Could you check a few things on this model? Use its own coordinates, in mm. Face numbers are marked on the shaded views. A direction names the side the tool comes from. Coordinates: 2 decimals unless noted, no trailing zeros. Loops run counter-clockwise (first coordinate to the right, second up) from the corner with the lowest first, then second, coordinate; pieces in that order, holes last.
from build123d import *

# Parameters (mm, degrees)
SKETCH001_R   = 8.9
SKETCH001_R_2 = 7.9
PAD001_DEPTH  = 10
SKETCH002_W   = 2.5
SKETCH002_H   = 12
PAD002_DEPTH  = 2
SKETCH003_R   = 4.5
SKETCH003_R_2 = 3.5
PAD003_DEPTH  = 6
SKETCH004_R   = 1
POCKET_DEPTH  = 14.351


with BuildPart() as part:
    # Sketch001 → Pad001 (new body)
    with BuildSketch(Plane.XY):
        Circle(SKETCH001_R)
        Circle(SKETCH001_R_2, mode=Mode.SUBTRACT)
    extrude(amount=PAD001_DEPTH)

    # Sketch002 → Pad002 (join)
    with BuildSketch(Plane.XY):
        with BuildLine():
            Line((14.35, -8), (14.35, 8))
            Line((0, 8.9), (14.35, 8))
            ThreePointArc((0, 8.9), (-8.9, 0), (0, -8.9))
            Line((0, -8.9), (14.35, -8))
        make_face()
        with Locations((11.1, 0)):
            Rectangle(SKETCH002_W, SKETCH002_H, mode=Mode.SUBTRACT)
    extrude(amount=PAD002_DEPTH)

    # Sketch003 → Pad003 (join)
    with BuildSketch(Plane.XY):
        Circle(SKETCH003_R)
        Circle(SKETCH003_R_2, mode=Mode.SUBTRACT)
    extrude(amount=PAD003_DEPTH)

    # Sketch004 → Pocket (cut, through all)
    with BuildSketch(Plane.YZ):
        with Locations((0, 3.5)):
            Circle(SKETCH004_R)
    extrude(amount=POCKET_DEPTH, mode=Mode.SUBTRACT)


solid = part.part
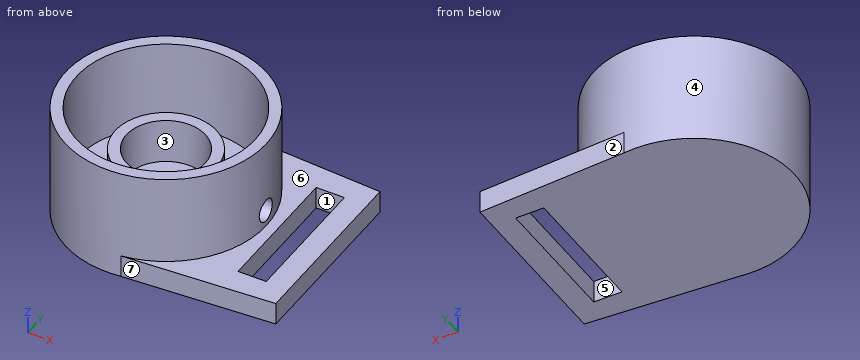
(1) Which directions (+Z, -Z, +X, -X, +Y, -Y) give clear straight access to the entire face, cutting with the end or side of a thin tool? Please do the marked faces 1, 2 and 3.
Answers:
face 1: +Z, -Z
face 2: +Z, -Z, +X, +Y
face 3: +Z
(2) Imagine slicing it at D-D, the plane y = 5.25. Write out the boundary of the cut face in (x, z).
Answers:
outline: (-7.19, 0) - (9.85, 0) - (9.85, 2) - (7.19, 2) - (7.19, 10) - (5.9, 10) - (5.9, 2) - (-5.9, 2) - (-5.9, 10) - (-7.19, 10) - close; (12.35, 0) - (14.35, 0) - (14.35, 2) - (12.35, 2) - close
(3) Imagine slicing it at A-A, the plane y = 0. State how many separate pieces and enclosed holes the cut face has, and give its area (3 significant figures).
Answers:
separate pieces: 4
enclosed holes: 0
area: 61.5 mm2
(4) I need wall thicknesses on probe 1 along X at (y, z) = (0, 5); probe 2 along Y at (x, z) = (-2.5, 5.25). Which ranges of each line are inside material? Lowest first, please.
Answers:
probe 1: x = -8.9 to -7.9, -4.5 to -3.5, 3.5 to 4.5, 7.9 to 8.9
probe 2: y = -8.54 to -7.49, -3.74 to -2.45, 2.45 to 3.74, 7.49 to 8.54
(5) Imagine slicing it at B-B, the plane z = 1.25. Write out the boundary of the cut face in (x, y), and give its area (3 significant figures).
Answers:
outline: (1.11, -8.83) - (14.35, -8) - (14.35, 8) - (1.11, 8.83) arc R8.9 ccw (long way) to start; hole (9.85, -6) - (12.35, -6) - (12.35, 6) - (9.85, 6) - close
area: 337 mm2
(6) Imagine slicing it at C-C, the plane x = 0. Write out the boundary of the cut face in (y, z), and give its area (3 significant figures).
Answers:
outline: (-8.9, 0) - (8.9, 0) - (8.9, 10) - (7.9, 10) - (7.9, 2) - (4.5, 2) - (4.5, 6) - (3.5, 6) - (3.5, 2) - (-3.5, 2) - (-3.5, 6) - (-4.5, 6) - (-4.5, 2) - (-7.9, 2) - (-7.9, 10) - (-8.9, 10) - close
area: 59.6 mm2
(7) For pin 1 (4 mm diameter, centred on x = 7.5, z = 3, fed in from +Y); pin 2 (4.5 mm diameter, centred on x = 2, y = -3.5, fed in from +Z); pin 3 (1.5 mm diameter, centred on x = -1.5, z = 1.5, fed in from +Y), each with a flat end and sliding along its axis, tell me the tip position at first contact or that it passes through.
Answers:
pin 1: stops at y = 8.54
pin 2: stops at z = 6
pin 3: stops at y = 8.87
(8) We'd pull the mould along X, two halves only. Please class the marked faces 4, 5, 6 and 7: +X half, -X half, draft (parallel to the pull), parting line (faces both ways), or undercut.
Answers:
face 4: parting line
face 5: undercut
face 6: draft
face 7: +X half
